Verification items for the finished model (mm, model axes). Coordinates: 2 decimals unless noted, no trailing zeros. Order: outer loops, then holes, each group sorted by start corner. A loop starts at its lowest first (then second) coordinate and runs counter-clockwise, first axis right, second up. Notation, with made-up numbers: M -39.75,-28.75 L -9.75,-28.75 A14 ccw -9.75,-23.75 Z; hole C -29.75,-2.75 d3. An arc over 180 degrees is marked long. Answer as a JSON object with one key per item and string values. Group by question number.
(1) Cross-section at D-D (z = -58). Enter the section's corners in (x, y).
(2) Cross-section at C-C (x = 69.85). Enter the section's corners in (y, z).
(3) Material ranges on line 1 (X direction, y = 23.5, z = -7.5); line 2 (X direction, y = 10.5, z = -61.5); line 3 (Y direction, x = 66.5, z = -35.5), recorded low to high.
(4) Cross-section at A-A (y = 21). Enter the section's corners in (x, z).
(5) Cross-section at B-B (z = 17.5). Enter the section's corners in (x, y).
from build123d import *

# Parameters (mm, degrees)
BOSS_EXTRUDE1_DEPTH = 76.2
FILLET1_R           = 25.4


with BuildPart() as part:
    # Sketch1 → Boss-Extrude1 (new, symmetric)
    with BuildSketch(Plane.XY):
        with BuildLine():
            Line((-152.4, 25.4), (-152.4, -25.4))
            Line((-152.4, -25.4), (152.4, -25.4))
            Line((152.4, -25.4), (152.4, 25.4))
            Line((152.4, 25.4), (95.25, 25.4))
            ThreePointArc((95.25, 25.4), (69.85, 0), (44.45, 25.4))
            Line((44.45, 25.4), (-44.45, 25.4))
            ThreePointArc((-44.45, 25.4), (-69.85, 0), (-95.25, 25.4))
            Line((-95.25, 25.4), (-152.4, 25.4))
        make_face()
    extrude(amount=BOSS_EXTRUDE1_DEPTH, both=True)

    # Fillet1
    fillet1_edges = [part.edges().sort_by_distance(p)[0] for p in [
        (-152.4, 0, -76.2),
        (-152.4, 0, 76.2),
        (152.4, 0, 76.2),
        (152.4, 0, -76.2),
    ]]
    fillet(fillet1_edges, radius=FILLET1_R)


solid = part.part
Taken from the geometry:
{
 "1": {"outline": "M -151.36,-25.4 L 151.36,-25.4 L 151.36,25.4 L 95.25,25.4 A25.4 cw 44.45,25.4 L -44.45,25.4 A25.4 cw -95.25,25.4 L -151.36,25.4 Z"},
 "2": {"outline": "M -25.4,-76.2 L 0,-76.2 L 0,76.2 L -25.4,76.2 Z"},
 "3": {"line 1": "x = -152.4 to -95.18, -44.52 to 44.52, 95.18 to 152.4", "line 2": "x = -150.04 to -90.42, -49.28 to 49.28, 90.42 to 150.04", "line 3": "y = -25.4 to 0.22"},
 "4": {"outline": "M -152.4,-50.8 A25.4 ccw -127,-76.2 L -94.87,-76.2 L -94.87,76.2 L -127,76.2 A25.4 ccw -152.4,50.8 Z; M -44.83,-76.2 L 44.83,-76.2 L 44.83,76.2 L -44.83,76.2 Z; M 94.87,-76.2 L 127,-76.2 A25.4 ccw 152.4,-50.8 L 152.4,50.8 A25.4 ccw 127,76.2 L 94.87,76.2 Z"},
 "5": {"outline": "M -152.4,-25.4 L 152.4,-25.4 L 152.4,25.4 L 95.25,25.4 A25.4 cw 44.45,25.4 L -44.45,25.4 A25.4 cw -95.25,25.4 L -152.4,25.4 Z"}
}
